from build123d import *

# Parameters (mm, degrees)
SKETCH1_W           = 59.055
SKETCH1_H           = 85.09
BOSS_EXTRUDE1_DEPTH = 4.7625
CUT_EXTRUDE1_REACH  = 203.148
SKETCH2_R           = 1.5875
CUT_EXTRUDE2_DEPTH  = 202.147856386
FILLET1_R           = 2.54


with BuildPart() as part:
    # Sketch1 → Boss-Extrude1 (new body)
    with BuildSketch(Plane(origin=(0, 0, 0), x_dir=(0, 0, -1), z_dir=(1, 0, 0))):
        with Locations((-162.318935185, 17.727083333)):
            Rectangle(SKETCH1_W, SKETCH1_H)
    extrude(amount=BOSS_EXTRUDE1_DEPTH)

    # Sketch2 → Cut-Extrude1 (cut, up to next)
    with BuildSketch(Plane(origin=(4.7625, 0, 0), x_dir=(0, 0, -1), z_dir=(1, 0, 0)), mode=Mode.PRIVATE) as cut_extrude1_sk1:
        with Locations((-188.466435185, -1.227916667)):
            Circle(SKETCH2_R)
    cut_extrude1_tool1 = extrude(cut_extrude1_sk1.sketch, amount=-CUT_EXTRUDE1_REACH, mode=Mode.PRIVATE) & part.part
    # Sketch2 → Cut-Extrude1 (cut, up to next)
    with BuildSketch(Plane(origin=(4.7625, 0, 0), x_dir=(0, 0, -1), z_dir=(1, 0, 0)), mode=Mode.PRIVATE) as cut_extrude1_sk2:
        with Locations((-139.466435185, -1.227916667)):
            Circle(SKETCH2_R)
    cut_extrude1_tool2 = extrude(cut_extrude1_sk2.sketch, amount=-CUT_EXTRUDE1_REACH, mode=Mode.PRIVATE) & part.part
    # Sketch2 → Cut-Extrude1 (cut, up to next)
    with BuildSketch(Plane(origin=(4.7625, 0, 0), x_dir=(0, 0, -1), z_dir=(1, 0, 0)), mode=Mode.PRIVATE) as cut_extrude1_sk3:
        with Locations((-139.466435185, 56.772083333)):
            Circle(SKETCH2_R)
    cut_extrude1_tool3 = extrude(cut_extrude1_sk3.sketch, amount=-CUT_EXTRUDE1_REACH, mode=Mode.PRIVATE) & part.part
    # Sketch2 → Cut-Extrude1 (cut, up to next)
    with BuildSketch(Plane(origin=(4.7625, 0, 0), x_dir=(0, 0, -1), z_dir=(1, 0, 0)), mode=Mode.PRIVATE) as cut_extrude1_sk4:
        with Locations((-188.466435185, 56.772083333)):
            Circle(SKETCH2_R)
    cut_extrude1_tool4 = extrude(cut_extrude1_sk4.sketch, amount=-CUT_EXTRUDE1_REACH, mode=Mode.PRIVATE) & part.part
    add(cut_extrude1_tool1.solids().sort_by_distance((4.7625, -1.227917, 188.466435))[0], mode=Mode.SUBTRACT)
    add(cut_extrude1_tool2.solids().sort_by_distance((4.7625, -1.227917, 139.466435))[0], mode=Mode.SUBTRACT)
    add(cut_extrude1_tool3.solids().sort_by_distance((4.7625, 56.772083, 139.466435))[0], mode=Mode.SUBTRACT)
    add(cut_extrude1_tool4.solids().sort_by_distance((4.7625, 56.772083, 188.466435))[0], mode=Mode.SUBTRACT)

    # Sketch3 → Cut-Extrude2 (cut, through all)
    with BuildSketch(Plane.ZY):
        Polygon((132.791435185, 47.572083333), (135.966435185, 47.572083333), (135.966435185, 48.397583333), (137.744435185, 48.397583333), (137.744435185, 47.572083333), (141.427435185, 47.572083333), (141.427435185, 44.270083333), (137.744435185, 44.270083333), (137.744435185, 43.444583333), (135.966435185, 43.444583333), (135.966435185, 44.270083333), (132.791435185, 44.270083333), align=None)
        Polygon((132.791435185, -8.307916667), (135.966435185, -8.307916667), (135.966435185, -7.482416667), (137.744435185, -7.482416667), (137.744435185, -8.307916667), (141.427435185, -8.307916667), (141.427435185, -11.609916667), (137.744435185, -11.609916667), (137.744435185, -12.435416667), (135.966435185, -12.435416667), (135.966435185, -11.609916667), (132.791435185, -11.609916667), align=None)
    extrude(amount=-CUT_EXTRUDE2_DEPTH, mode=Mode.SUBTRACT)

    # Fillet1
    fillet1_edges = [part.edges().sort_by_distance(p)[0] for p in [
        (2.38125, -24.817916667, 191.846435185),
        (2.38125, 60.272083333, 191.846435185),
    ]]
    fillet(fillet1_edges, radius=FILLET1_R)


solid = part.part
The listing builds one solid part. Answer for the finished solid, in the listing's coordinates (mm). A direction names the side the tool comes from. Round coordinates to 2 decimals unless told otherwise and drop trailing zeros. Order: outer loops, then holes, each group sorted by start corner. A loop starts at its lowest first (then second) coordinate and runs counter-clockwise, first axis right, second up. Notation, with made-up numbers: (-23, 76) - (4, 76) arc R31 cw to (4, 103) - close; hole circle Ø10 at (87.25, -37). An arc over 180 degrees is marked (long way). Write item = value, one per line. Start each with the question number.
1) For a pull along Y with two mould halves and no side action, classify faces 4 (the flat face through (2, 47.572, 134)), 5 (the flat face through (4.762, 18, 163)), 6 (the cylindrical face through (2.415, -24.054, 191.122)), 7 (the flat face through (2, 47.572, 140)) as released by +Y, released by -Y, zero draft, split by the parting line, or undercut.
2) Straight lines are drawn through the part: L1, parallel to Z at x = 3.2, y = -8; L2, parallel to Y at x = 2.9, z = 140; L3, parallel to Z at x = 1, y = -8.5. For each, find the intervals that lie inside material, in ascending order.
3) Section B-B, the plane y = -9.5 is taken. Write down the section's boundary in (x, z).
4) Section A-A, the plane x = 3.35 is taken. Count the separate pieces of the cut face and the enclosed holes in it, plus the area to 3 significant figures.
5) For faces 1 (the flat face through (2, 46, 141.427)), 2 (the flat face through (2, -18, 132.791)), 3 (the flat face through (2, 48.398, 137)), determine the directions among +Z, -Z, +X, -X, +Y, -Y from which every point of the face is accessible in a straight line to the end or side of a thin tool.
6) Given pin 1 (1 mm diameter, centred on x = 1.5, y = 46, fed in from -Z); pin 2 (3 mm diameter, centred on y = 56.77, z = 139.47, fed in from -X), each flat-ended and moving along its own axis, determine where each tip first touches the part or whether it passes through.
Results list:
q1.face_4 = undercut
q1.face_5 = zero draft
q1.face_6 = released by -Y
q1.face_7 = undercut
q2.L1 = 132.79 to 135.97, 137.74 to 191.85
q2.L2 = -24.82 to -11.61, -8.31 to -2.72, 0.27 to 44.27, 47.57 to 55.28, 58.27 to 60.27
q2.L3 = 141.43 to 191.85
q3.outline = (0, 141.43) - (4.76, 141.43) - (4.76, 191.85) - (0, 191.85) - close
q4.separate_pieces = 1
q4.enclosed_holes = 4
q4.area = 4,930 mm^2
q5.face_1 = -Z, +X, -X
q5.face_2 = -Z, +X, -X, +Y, -Y
q5.face_3 = +X, -X
q6.pin_1 = 141.43
q6.pin_2 = through
